from build123d import *

# Parameters (mm, degrees)
SKETCH1_R                = 5.04
BOSS_EXTRUDE1_DEPTH      = 15
CUT_EXTRUDE1_DEPTH       = 15
FILLET2_R                = 0.43
CIRPATTERN1_COUNT        = 5
FILLET2_OF_CIRPATTERN1_R = 0.43


with BuildPart() as part:
    # Sketch1 → Boss-Extrude1 (new body, symmetric)
    with BuildSketch(Plane(origin=(0, 0, 0), x_dir=(1, 0, 0), z_dir=(0, 1, 0))):
        Circle(SKETCH1_R)
    extrude(amount=BOSS_EXTRUDE1_DEPTH, both=True)

    # Sketch2 → Cut-Extrude1 (cut, symmetric)
    with BuildSketch(Plane(origin=(0, 0, 0), x_dir=(1, 0, 0), z_dir=(0, 1, 0))):
        with BuildLine():
            ThreePointArc((-1.594286027, 4.781197764), (-1.02324782, 3.327591934), (-0.539761549, 1.842568173))
            ThreePointArc((-0.539761549, 1.842568173), (0, 1.92), (0.539761549, 1.842568173))
            ThreePointArc((0.539761549, 1.842568173), (1.02324782, 3.327591934), (1.594286027, 4.781197764))
            ThreePointArc((1.594286027, 4.781197764), (0, 5.04), (-1.594286027, 4.781197764))
        make_face()
    cut_extrude1 = extrude(amount=CUT_EXTRUDE1_DEPTH, both=True, mode=Mode.SUBTRACT)

    # Fillet2
    fillet2_edges = [part.edges().sort_by_distance(p)[0] for p in [
        (0.539761549, 0, -1.842568173),
        (-0.539761549, 0, -1.842568173),
    ]]
    fillet(fillet2_edges, radius=FILLET2_R)

    # CirPattern1: Cut-Extrude1 ×5 about axis
    cirpattern1_axis = Axis((0, 0, 0), (0, 1, 0))
    for i in range(1, CIRPATTERN1_COUNT):
        add(cut_extrude1.rotate(cirpattern1_axis, i * 360 / CIRPATTERN1_COUNT), mode=Mode.SUBTRACT)

    # Fillet2 of CirPattern1
    fillet2_of_cirpattern1_edges = [part.edges().sort_by_distance(p)[0] for p in [
        (-1.585590976, 0, -1.082728617),
        (-1.919181959, 0, -0.05604114),
        (-1.519710664, 0, 1.173405087),
        (-0.646358132, 0, 1.807932843),
        (0.646358132, 0, 1.807932843),
        (1.519710664, 0, 1.173405087),
        (1.919181959, 0, -0.05604114),
        (1.585590976, 0, -1.082728617),
    ]]
    fillet(fillet2_of_cirpattern1_edges, radius=FILLET2_OF_CIRPATTERN1_R)


solid = part.part
CAD build for the part. Positions are in the model's coordinates, mm. A direction names the side the tool comes from. Round coordinates to 2 decimals unless told otherwise and drop trailing zeros. Write each loop counter-clockwise with the first axis right and the second up, starting at its lowest first coordinate (ties: lowest second). Pieces come first, ordered by that corner, then holes.
(1) Probe line 1 along X through (y, z) = (-3, 1.75); line 2 along X through (y, z) = (-5.5, 2.75); line 3 along Z through (x, y) = (3.5, -6). List the from-to ranges inside material, lowest first.
(2) Mould opens along Z. For faces 5 (the face through (2.98, 0.21, -4.065)), 6 (the face through (-2.99, 0.21, -2.11)), 7 (the face through (-4.8, 0.21, 1.54)) say: pulls with the +Z half, pulls with the -Z half, needs draft (parallel to the pull), parting line crosses it, or undercut.
(3) Slice it at B-B, the plane z = 1. Write the cut outline in (x, y).
(4) 3-axis set-ups, long thin cutter, end or side, ignore diameter. For faces 1 (the face through (3.015, 0.21, -2.132)), 2 (the face through (1.082, 0.21, -3.49)), 3 (the face through (1.176, 0.21, 3.46)), 4 (the face through (-2.93, 0.21, 2.19)): which of +Z, -Z, +X, -X, +Y, -Y reach the whole face in a straight line?
(5) Slice it at A-A, the plane x = -3.75. Write the cut outline in (y, z), and give its area (3 significant figures).
(6) Drop flat-ended pins along their axis: P1, Ø3, axis at y = -11, z = 2.5, coming from the +X side; P2, Ø4, axis at y = 3, z = 2.5, coming from the -X side; P3, Ø1.5, axis at y = 3, z = -2, coming from the -X side. Give the stop position or say it passes through.
From the geometry:
1. line 1: x = -4.73 to -2.3, -0.86 to 0.86, 2.3 to 4.73
1. line 2: x = -4.22 to -3.8, -0.96 to 0.96, 3.8 to 4.22
1. line 3: z = -3.63 to -2.52, -0.05 to 2.56
2. face 5: pulls with the -Z half
2. face 6: undercut
2. face 7: pulls with the +Z half
3. outline: (-4.94, -15) - (4.94, -15) - (4.94, 15) - (-4.94, 15) - close
4. face 1: +X, +Y, -Y
4. face 2: -Z, +Y, -Y
4. face 3: +Y, -Y
4. face 4: +Z, +Y, -Y
5. outline: (-15, -3.37) - (15, -3.37) - (15, -2.73) - (-15, -2.73) - close; (-15, -0.05) - (15, -0.05) - (15, 2.72) - (-15, 2.72) - close
5. area: 102 mm2
6. P1: stops at x = 4.94
6. P2: stops at x = -5.02
6. P3: stops at x = -3.77
